from build123d import *

# Parameters (mm, degrees)
PAD_DEPTH         = 7
SKETCH001_R       = 4.25
PAD001_DEPTH      = 20
PAD001_DEPTH_BACK = 10


with BuildPart() as part:
    # Sketch → Pad (new body)
    with BuildSketch(Plane.XY):
        Polygon((0, -7.794229), (6.75, -3.897114), (6.75, 3.897114), (0, 7.794229), (-6.75, 3.897114), (-6.75, -3.897114), align=None)
    extrude(amount=PAD_DEPTH)

    # Sketch001 → Pad001 (join, two sides)
    with BuildSketch(Plane.XY) as pad001_sk:
        Circle(SKETCH001_R)
    extrude(amount=PAD001_DEPTH)
    extrude(pad001_sk.sketch, amount=-PAD001_DEPTH_BACK)


solid = part.part
Work out the finished part from the listing and answer in its coordinate system (mm). A direction names the side the tool comes from. Round coordinates to 2 decimals unless told otherwise and drop trailing zeros. Write each loop counter-clockwise with the first axis right and the second up, starting at its lowest first coordinate (ties: lowest second). Pieces come first, ordered by that corner, then holes. Notation, with made-up numbers: M 63.25,-30 L 83.25,-30 A25 cw 83.25,-10 Z; hole C 4,46.5 d11. An arc over 180 degrees is marked long. Use a Markdown table: item, result.
1) The part is cut by section D-D on y = 5.75. Give the vertices of the cut face in (x, z), plus the area to 3 significant figures.
Taken from the geometry:
| item | result |
|---|---|
| outline | M -3.54,0 L 3.54,0 L 3.54,7 L -3.54,7 Z |
| area | 49.6 mm2 |
2) Flat-ended cylindrical pins translate along their axes: pin 1 (2 mm diameter, centred on y = -1.5, z = 12.5, fed in from -X); pin 2 (1.5 mm diameter, centred on y = -3, z = -5.5, fed in from -X); pin 3 (8 mm diameter, centred on x = -4.5, z = 5.5, fed in from -Y). Find the tip coordinate at first contact, or state that the pin passes through.
Taken from the geometry:
| item | result |
|---|---|
| pin 1 | stops at x = -4.22 |
| pin 2 | stops at x = -3.61 |
| pin 3 | stops at y = -7.51 |
3) The part is cut by section A-A on x = -1.5. Give the vertices of the cut face in (y, z).
Taken from the geometry:
| item | result |
|---|---|
| outline | M -6.93,0 L -3.98,0 L -3.98,-10 L 3.98,-10 L 3.98,0 L 6.93,0 L 6.93,7 L 3.98,7 L 3.98,20 L -3.98,20 L -3.98,7 L -6.93,7 Z |
4) The part is cut by section C-C on z = -5.5. Give the vertices of the cut face in (x, y).
Taken from the geometry:
| item | result |
|---|---|
| outline | C 0,0 d8.5 |
5) Consider line 1 (Z direction, x = 0.5, y = 6); line 2 (X direction, y = 0.25, z = 8.25); line 3 (X direction, y = 1.25, z = -7.75). Determine where each line is inside the solid, lowest interval first. Write a range as [from, to].
Taken from the geometry:
| item | result |
|---|---|
| line 1 | z = [0, 7] |
| line 2 | x = [-4.24, 4.24] |
| line 3 | x = [-4.06, 4.06] |
6) The part is cut by section B-B on y = 0. Give the vertices of the cut face in (x, z), plus the area to 3 significant figures.
Taken from the geometry:
| item | result |
|---|---|
| outline | M -6.75,0 L -4.25,0 L -4.25,-10 L 4.25,-10 L 4.25,0 L 6.75,0 L 6.75,7 L 4.25,7 L 4.25,20 L -4.25,20 L -4.25,7 L -6.75,7 Z |
| area | 290 mm2 |
7) Determine the mould class of faces 1 (the face through (0, 0, -10)), 2 (the face through (2.9, -3.4, 7)), 3 (the face through (-3.33, 5.87, 3.45)) for opening direction Z: pulls with the +Z half, pulls with the -Z half, needs draft (parallel to the pull), parting line crosses it, or undercut.
Taken from the geometry:
| item | result |
|---|---|
| face 1 | pulls with the -Z half |
| face 2 | pulls with the +Z half |
| face 3 | needs draft |
8) Which of the six approach directions +Z, -Z, +X, -X, +Y, -Y give full straight-line access (tool end or side, diameter ignored) to faces 4 (the face through (2.285, 3.584, -4.93)), 5 (the face through (-6.75, 0, 3)), 6 (the face through (2.285, 3.584, 13.409))?
Taken from the geometry:
| item | result |
|---|---|
| face 4 | -Z |
| face 5 | +Z, -Z, -X, +Y, -Y |
| face 6 | +Z |
